Build history of the part. All positions in model axes, mm. A direction names the side the tool comes from. Round coordinates to 2 decimals unless told otherwise and drop trailing zeros. Order: outer loops, then holes, each group sorted by start corner. A loop starts at its lowest first (then second) coordinate and runs counter-clockwise, first axis right, second up. Notation, with made-up numbers: (62.25, 88) -> (83.25, 88) arc R23 cw to (83.25, 103) -> close; hole circle Ø3 at (14.25, 84.5). An arc over 180 degrees is marked (long way). Answer as a JSON object with one key per item and string values.
from build123d import *
from build123d.topology import SkipClean

# Parameters (mm, degrees)
MAIN_DEPTH                                        = 3
R_P_TITION_CIRCULAIRE1_COUNT                      = 8
ESQUISSE2_R                                       = 8.925
ESQUISSE2_R_2                                     = 3.1
MOTORLINK_DEPTH                                   = 10
MEPLAT_DEPTH                                      = 10
ESQUISSE4_R                                       = 3.1
HOLE_DEPTH                                        = 29.670542374
ESQUISSE5_R                                       = 4
ESQUISSE5_R_2                                     = 3.1
ROLLINGBEARINGLINK_DEPTH                          = 7
ESQUISSE6_R                                       = 5
ESQUISSE6_R_2                                     = 4
ROLLINGBEARLINK2_DEPTH                            = 0.5
FRAISAGE_POUR_VIS_T_TE_FRAIS_E_100_D              = 3.2
FRAISAGE_POUR_VIS_T_TE_FRAIS_E_100_CSINK_D        = 5.5
FRAISAGE_POUR_VIS_T_TE_FRAIS_E_100_CSINK_ANGLE    = 100
R_P_TITION_CIRCULAIRE2_COUNT                      = 8
CSK_FOR_M2_5_FLAT_HEAD_MACHINE_SCREW1_D           = 2.9
CSK_FOR_M2_5_FLAT_HEAD_MACHINE_SCREW1_CSINK_D     = 5.5
CSK_FOR_M2_5_FLAT_HEAD_MACHINE_SCREW1_CSINK_ANGLE = 90


with BuildPart() as part:
    # Esquisse1 → Main (new body)
    with BuildSketch(Plane.XY):
        with BuildLine():
            Line((11.313708499, 4), (15, 4))
            ThreePointArc((15, 4), (19, 0), (15, -4))
            Line((15, -4), (11.313708499, -4))
            ThreePointArc((11.313708499, -4), (11.204044803, -4.297601664), (11.08655439, -4.592201188))
            Line((11.08655439, -4.592201188), (0, 0))
            Line((0, 0), (11.08655439, 4.592201188))
            ThreePointArc((11.08655439, 4.592201188), (11.204044803, 4.297601664), (11.313708499, 4))
        make_face()
    main = extrude(amount=MAIN_DEPTH)

    # R_p_tition circulaire1: Main ×8 about axis
    r_p_tition_circulaire1_axis = Axis((0, 0, 0), (0, 0, 1))
    for i in range(1, R_P_TITION_CIRCULAIRE1_COUNT):
        add(main.rotate(r_p_tition_circulaire1_axis, i * 360 / R_P_TITION_CIRCULAIRE1_COUNT))

    # Esquisse2 → MotorLink (add)
    with BuildSketch(Plane.XY.offset(3)):
        with Locations(Location((0, 0, 0), (0, 0, 180))):
            Circle(ESQUISSE2_R)
        Circle(ESQUISSE2_R_2, mode=Mode.SUBTRACT)
    extrude(amount=MOTORLINK_DEPTH)

    # Esquisse3 → Meplat (add)
    with BuildSketch(Plane.XY.offset(3)):
        with BuildLine():
            Line((-2.368543856, 2), (2.368543856, 2))
            ThreePointArc((2.368543856, 2), (0, 3.1), (-2.368543856, 2))
        make_face()
    extrude(amount=MEPLAT_DEPTH)

    # Esquisse4 → Hole (cut, through all)
    with SkipClean():  # the faces are left unmerged after this step: merging them gives an invalid solid
        with BuildSketch(Plane.XY.offset(3)):
            with Locations(Location((0, 0, 0), (0, 0, 139.82223046))):
                Circle(ESQUISSE4_R)
        extrude(amount=-HOLE_DEPTH, mode=Mode.SUBTRACT)

    # Esquisse5 → RollingBearingLink (add)
    with SkipClean():  # the faces are left unmerged after this step: merging them gives an invalid solid
        with BuildSketch(Plane(origin=(0, 0, 0), x_dir=(-1, 0, 0), z_dir=(0, 0, -1))):
            Circle(ESQUISSE5_R)
            Circle(ESQUISSE5_R_2, mode=Mode.SUBTRACT)
        extrude(amount=ROLLINGBEARINGLINK_DEPTH)

    # Esquisse6 → RollingBearLink2 (add)
    with SkipClean():  # the faces are left unmerged after this step: merging them gives an invalid solid
        with BuildSketch(Plane(origin=(0, 0, 0), x_dir=(-1, 0, 0), z_dir=(0, 0, -1))):
            Circle(ESQUISSE6_R)
            Circle(ESQUISSE6_R_2, mode=Mode.SUBTRACT)
        extrude(amount=ROLLINGBEARLINK2_DEPTH)
    add(part.part.scale(1), mode=Mode.REPLACE)  # the faces are merged on a copy

    # Fraisage pour vis _ t_te frais_e _100 (through all)
    with Locations(Plane(origin=(0, 0, 0), x_dir=(-1, 0, 0), z_dir=(0, 0, -1))):
        with Locations((15, 0)):
            fraisage_pour_vis_t_te_frais_e_100 = CounterSinkHole(FRAISAGE_POUR_VIS_T_TE_FRAIS_E_100_D / 2, FRAISAGE_POUR_VIS_T_TE_FRAIS_E_100_CSINK_D / 2, counter_sink_angle=FRAISAGE_POUR_VIS_T_TE_FRAIS_E_100_CSINK_ANGLE)

    # R_p_tition circulaire2: Fraisage pour vis _ t_te frais_e _100 ×8 about axis
    r_p_tition_circulaire2_axis = Axis((0, 0, 0), (0, 0, 1))
    for i in range(1, R_P_TITION_CIRCULAIRE2_COUNT):
        add(fraisage_pour_vis_t_te_frais_e_100.rotate(r_p_tition_circulaire2_axis, i * 360 / R_P_TITION_CIRCULAIRE2_COUNT), mode=Mode.SUBTRACT)

    # CSK for M2.5 Flat Head Machine Screw1 (through all)
    with Locations(Plane(origin=(0, 8.925, 0), x_dir=(1, 0, 0), z_dir=(0, 1, 0))):
        with Locations((0, -8)):
            CounterSinkHole(CSK_FOR_M2_5_FLAT_HEAD_MACHINE_SCREW1_D / 2, CSK_FOR_M2_5_FLAT_HEAD_MACHINE_SCREW1_CSINK_D / 2, counter_sink_angle=CSK_FOR_M2_5_FLAT_HEAD_MACHINE_SCREW1_CSINK_ANGLE)


solid = part.part
1) Flat gauge pins, fed straight in: pin 1 Ø1.5 at (y, z) = (-2, 0) entering from -X; pin 2 Ø3 at (x, y) = (15, 0) entering from +Z; pin 3 Ø2.5 at (x, z) = (-13, 1.5) entering from +Y; pin 4 Ø2.5 at (y, z) = (-14, 1.5) entering from +X. Where does each tip first touch, or does it go through?
Checked values:
{"pin 1": "stops at x = -18.8", "pin 2": "passes through", "pin 3": "stops at y = 14.44", "pin 4": "stops at x = 13.98"}
2) Cut at A-A, the plane z = -4.75. Give the cut face in (x, y), plus the area to 3 significant figures.
Checked values:
{"outline": "circle Ø8 at (0, 0); hole circle Ø6.2 at (0, 0)", "area": "20.1 mm²"}
3) Cut at B-B, the plane x = 0. Count the separate pieces of the cut face and the enclosed holes in it, plus the area to 3 significant figures.
Checked values:
{"separate pieces": "6", "enclosed holes": "0", "area": "176 mm²"}
4) Which spindle directions (+Z, -Z, +X, -X, +Y, -Y) get a long thin tool onto all of the face, cutting with end or side? Do faces 1 (the face through (-4, -13, 1)), 2 (the face through (-4, 13, 1)), 3 (the face through (-13, -4, 1)). Say none if no direction does.
Checked values:
{"face 1": "+Z, -Z, -Y", "face 2": "+Z, -Z, +Y", "face 3": "+Z, -Z, -X"}
5) Cut at D-D, the plane x = 6. Give the cut face in (y, z), plus the area to 3 significant figures.
Checked values:
{"outline": "(-11.66, 0) -> (11.66, 0) -> (11.66, 3) -> (6.61, 3) -> (6.61, 13) -> (-6.61, 13) -> (-6.61, 3) -> (-11.66, 3) -> close", "area": "202 mm²"}
6) Cut at C-C, the plane y = -6. Give the cut face in (x, z), plus the area to 3 significant figures.
Checked values:
{"outline": "(-11.66, 0) -> (11.66, 0) -> (11.66, 3) -> (6.61, 3) -> (6.61, 13) -> (-6.61, 13) -> (-6.61, 3) -> (-11.66, 3) -> close; hole circle Ø2.9 at (0, 8)", "area": "195 mm²"}
7) Probe L1, parallel to X at y = 0, z = 1.85; L2, parallel to Y at x = -15, z = 1.9. List the from-to ranges inside material, lowest first. Write a range as from..to.
Checked values:
{"L1": "x = -19..-16.6, -13.4..-3.1, 3.1..13.4, 16.6..19", "L2": "y = -4..-1.6, 1.6..4"}
